from build123d import *

# Parameters (mm, degrees)
F0_W     = 15
F0_H     = 4
F1_DEPTH = 4
F2_DEPTH = 2
F3_DEPTH = 3.05
F4_DEPTH = 3.05


with BuildPart() as f1:
    # F0 (on Top) → F1 (new body)
    with BuildSketch(Plane.XY):
        Rectangle(F0_W, F0_H)
        Polygon((-4.3586225185, -1.525), (-7, 0), (-4.3586225185, 1.525), align=None, mode=Mode.SUBTRACT)
        Polygon((4.3586225185, 1.525), (7, 0), (4.3586225185, -1.525), align=None, mode=Mode.SUBTRACT)
    extrude(amount=F1_DEPTH)

    # F0 (on Top) → F2 (join)
    with BuildSketch(Plane.XY):
        Rectangle(F0_W, F0_H)
        Polygon((-4.3586225185, -1.525), (-7, 0), (-4.3586225185, 1.525), align=None, mode=Mode.SUBTRACT)
        Polygon((4.3586225185, 1.525), (7, 0), (4.3586225185, -1.525), align=None, mode=Mode.SUBTRACT)
        Polygon((-4.3586225185, 1.525), (-7, 0), (-4.3586225185, -1.525), align=None)
        Polygon((4.3586225185, -1.525), (7, 0), (4.3586225185, 1.525), align=None)
    extrude(amount=-F2_DEPTH)

    # F3 (cut): a face of the model
    f3_faces = [f1.faces().sort_by_distance(p)[0] for p in [
        (4.3586225185, 0, 2),
    ]]
    extrude(f3_faces, amount=-F3_DEPTH, mode=Mode.SUBTRACT)

    # F4 (cut): a face of the model
    f4_faces = [f1.faces().sort_by_distance(p)[0] for p in [
        (-4.3586225185, 0, 2),
    ]]
    extrude(f4_faces, amount=-F4_DEPTH, mode=Mode.SUBTRACT)


solid = f1.part
Build history of the part. All positions in model axes, mm. A direction names the side the tool comes from. Coordinates: 2 decimals unless noted, no trailing zeros. Write each loop counter-clockwise with the first axis right and the second up, starting at its lowest first coordinate (ties: lowest second). Pieces come first, ordered by that corner, then holes. Notation, with made-up numbers: (32, 17.25) -> (79, 17.25) arc R32 cw to (79, 49.25) -> close; hole circle Ø11 at (54.5, 73). An arc over 180 degrees is marked (long way). Use CSV: the item, a comma, the result in double quotes. Start each with the question number.
Q1. Pull direction Y, two halves, no side cores. Call faces 3 (the flat face through (0, -2, 1)), 4 (the flat face through (-4, 0, 0)), 5 (the flat face through (3, -1.525, 2)), 6 (the flat face through (0, 0, -2)): released by +Y, released by -Y, zero draft, split by the parting line, or undercut.
Q2. Cut at A-A, the plane z = 3.35. List the corners of the cut face in (x, y) (3 decimals).
Q3. Cut at C-C, the plane y = -0.7. List the corners of the cut face in (x, z), then the cut area to 3 significant figures.
Q4. Cut at D-D, the plane x = 5.75. List the corners of the cut face in (y, z).
Q5. 3-axis set-ups, long thin cutter, end or side, ignore diameter. For faces 1 (the flat face through (0, 2, 1)), 2 (the flat face through (3, 0, 0)): which of +Z, -Z, +X, -X, +Y, -Y reach the whole face in a straight line?
Q6. Cut at B-B, the plane x = 3.5. List the corners of the cut face in (y, z) (3 decimals), then the cut area to 3 significant figures.
Q7. Drill centre lines: probe 1 along X at (y, z) = (1.45, 1.35); probe 2 along Y at (x, z) = (-3.25, 2.7) (3 decimals); probe 3 along X at (y, z) = (0.1, 1.1). Where is each one in solid material? Low to high.
Checked values:
1,face 3,"released by -Y"
1,face 4,"undercut"
1,face 5,"undercut"
1,face 6,"zero draft"
2,outline,"(-7.5, -2) -> (7.5, -2) -> (7.5, 2) -> (-7.5, 2) -> close; hole (-7, 0) -> (-4.359, -1.525) -> (-1.309, -1.525) -> (-1.309, 1.525) -> (-4.359, 1.525) -> close; hole (1.309, -1.525) -> (4.359, -1.525) -> (7, 0) -> (4.359, 1.525) -> (1.309, 1.525) -> close"
3,outline,"(-7.5, -2) -> (7.5, -2) -> (7.5, 4) -> (5.79, 4) -> (5.79, 0) -> (1.31, 0) -> (1.31, 4) -> (-1.31, 4) -> (-1.31, 0) -> (-5.79, 0) -> (-5.79, 4) -> (-7.5, 4) -> close"
3,area,"54.2 mm²"
4,outline,"(-2, -2) -> (2, -2) -> (2, 4) -> (0.72, 4) -> (0.72, 0) -> (-0.72, 0) -> (-0.72, 4) -> (-2, 4) -> close"
5,face 1,"+Z, -Z, +X, -X, +Y"
5,face 2,"+Z"
6,outline,"(-2, -2) -> (2, -2) -> (2, 4) -> (1.525, 4) -> (1.525, 0) -> (-1.525, 0) -> (-1.525, 4) -> (-2, 4) -> close"
6,area,"11.8 mm²"
7,probe 1,"x = -7.5 to -4.49, -1.31 to 1.31, 4.49 to 7.5"
7,probe 2,"y = -2 to -1.525, 1.525 to 2"
7,probe 3,"x = -7.5 to -6.83, -1.31 to 1.31, 6.83 to 7.5"
